Geometry check sheet. Reference: the model listing, model coordinates, mm. Face numbers are marked on the shaded views. Round coordinates to 2 decimals unless told otherwise and drop trailing zeros. Write each loop counter-clockwise with the first axis right and the second up, starting at its lowest first coordinate (ties: lowest second). Pieces come first, ordered by that corner, then holes. Notation, with made-up numbers: (72, -34.75) -> (87, -34.75) arc R23 ccw to (87, -23.75) -> close; hole circle Ø6 at (-38.75, 87.5). An arc over 180 degrees is marked (long way). Put each result on its own line as item: value. Start each with the question number.
from build123d import *

# Parameters (mm, degrees)
CROQUIS1_W              = 1000
CROQUIS1_H              = 1000
SALIENTE_EXTRUIR1_DEPTH = 3.175
CROQUIS2_W              = 1000
CROQUIS2_H              = 1000
CROQUIS2_W_2            = 923.8
CROQUIS2_H_2            = 923.8
SALIENTE_EXTRUIR2_DEPTH = 38.1
CROQUIS3_W              = 38.1
CROQUIS3_H              = 38.1
SALIENTE_EXTRUIR3_DEPTH = 170
CROQUIS4_W              = 100
CROQUIS4_H              = 100
SALIENTE_EXTRUIR4_DEPTH = 3.175


with BuildPart() as part:
    # Croquis1 → Saliente-Extruir1 (new body)
    with BuildSketch(Plane(origin=(0, 0, 0), x_dir=(1, 0, 0), z_dir=(0, 1, 0))):
        Rectangle(CROQUIS1_W, CROQUIS1_H)
    extrude(amount=SALIENTE_EXTRUIR1_DEPTH)

    # Croquis2 → Saliente-Extruir2 (add)
    with BuildSketch(Plane(origin=(0, 0, 0), x_dir=(-1, 0, 0), z_dir=(0, -1, 0))):
        Rectangle(CROQUIS2_W, CROQUIS2_H)
        Rectangle(CROQUIS2_W_2, CROQUIS2_H_2, mode=Mode.SUBTRACT)
    extrude(amount=SALIENTE_EXTRUIR2_DEPTH)

    # Croquis3 → Saliente-Extruir3 (add)
    with BuildSketch(Plane.XZ.offset(38.1)):
        with Locations((480.95, 480.95)):
            Rectangle(CROQUIS3_W, CROQUIS3_H)
        with Locations((-480.95, 480.95)):
            Rectangle(CROQUIS3_W, CROQUIS3_H)
        with Locations((480.95, -480.95)):
            Rectangle(CROQUIS3_W, CROQUIS3_H)
        with Locations((-480.95, -480.95)):
            Rectangle(CROQUIS3_W, CROQUIS3_H)
    extrude(amount=SALIENTE_EXTRUIR3_DEPTH)

    # Croquis4 → Saliente-Extruir4 (add)
    with BuildSketch(Plane.XZ.offset(208.1)):
        with Locations((480.95, 480.95)):
            Rectangle(CROQUIS4_W, CROQUIS4_H)
        with Locations((-480.95, 480.95)):
            Rectangle(CROQUIS4_W, CROQUIS4_H)
        with Locations((480.95, -480.95)):
            Rectangle(CROQUIS4_W, CROQUIS4_H)
        with Locations((-480.95, -480.95)):
            Rectangle(CROQUIS4_W, CROQUIS4_H)
    extrude(amount=SALIENTE_EXTRUIR4_DEPTH)


solid = part.part
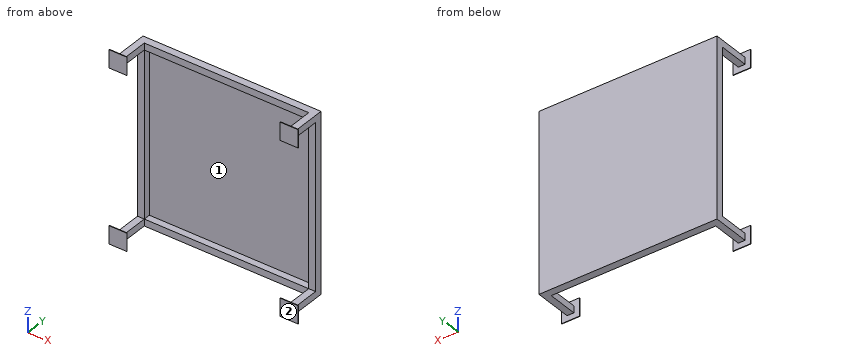
(1) Mould release check, pull along Z, two halves, no side actions. Record for the marked faces 1 and 2: +Z half, -Z half, draft (parallel to the pull), parting line (faces both ways), or undercut.
(2) Material ranges on L1, parallel to X at y = -89, z = 487.5; L2, parallel to Y at x = -425.5, z = -451.5 (3 decimals), recorded low to high. Write a range as from..to.
(3) Sectioned sample at B-B (z = -11). Record the cut outline in (x, y) (3 decimals).
(4) Go/stop test with flat-tipped pins: pin 1 Ø11.5 at (y, z) = (-98, -488.5) entering from +X; pin 2 Ø6 at (x, z) = (18, 17.5) entering from -Y; pin 3 Ø19 at (x, z) = (23, -487.5) entering from -Y. Record where each tip stops, or that it passes through.
(5) Sectioned sample at A-A (y = -156.5). Record the cut outline in (x, z), and give its area (3 significant figures).
(6) Sectioned sample at C-C (x = -108). Record the cut outline in (y, z) (3 decimals), and give its area (3 significant figures).
Found:
1. face 1: undercut
1. face 2: draft
2. L1: -500..-461.9, 461.9..500
2. L2: 0..3.175
3. outline: (-500, -38.1) -> (-461.9, -38.1) -> (-461.9, 0) -> (461.9, 0) -> (461.9, -38.1) -> (500, -38.1) -> (500, 3.175) -> (-500, 3.175) -> close
4. pin 1: x = 500
4. pin 2: y = 0
4. pin 3: y = -38.1
5. outline: (-500, -500) -> (-461.9, -500) -> (-461.9, -461.9) -> (-500, -461.9) -> close; (-500, 461.9) -> (-461.9, 461.9) -> (-461.9, 500) -> (-500, 500) -> close; (461.9, -500) -> (500, -500) -> (500, -461.9) -> (461.9, -461.9) -> close; (461.9, 461.9) -> (500, 461.9) -> (500, 500) -> (461.9, 500) -> close
5. area: 5,810 mm2
6. outline: (-38.1, -500) -> (3.175, -500) -> (3.175, 500) -> (-38.1, 500) -> (-38.1, 461.9) -> (0, 461.9) -> (0, -461.9) -> (-38.1, -461.9) -> close
6. area: 6,080 mm2
